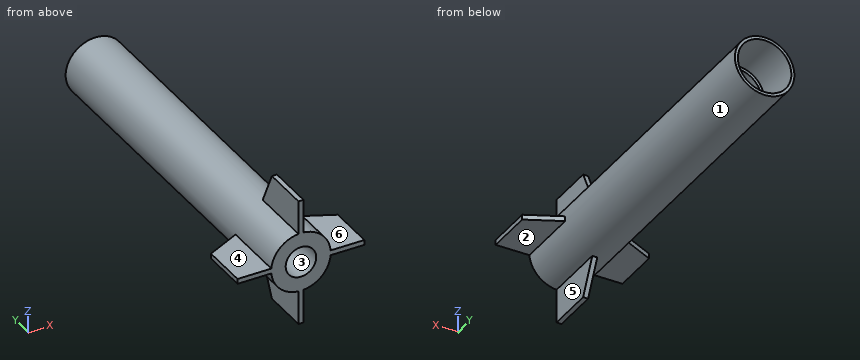
```python
from build123d import *

# Parameters (mm, degrees)
SKETCH1_R                = 11.925
SKETCH1_R_2              = 9.525
BOSS_EXTRUDE1_DEPTH      = 145
BOSS_EXTRUDE2_DEPTH      = 1
CIRPATTERN1_COUNT        = 4
SKETCH3_R                = 7.325
SKETCH3_R_2              = 6.125
BOSS_EXTRUDE3_DEPTH      = 87.75
CUT_EXTRUDE1_START       = -19
SKETCH4_R                = 10.725
SKETCH4_R_2              = 9.525
CUT_EXTRUDE1_DEPTH       = 19
BOSS_EXTRUDE4_START      = -1
SKETCH5_R                = 9.525
SKETCH5_R_2              = 6.125
BOSS_EXTRUDE4_DEPTH      = 1
BOSS_EXTRUDE5_DEPTH      = 0.5
BOSS_EXTRUDE5_DEPTH_BACK = 0.5
SKETCH6_R                = 9.525
SKETCH6_R_2              = 6.125
SKETCH7_R                = 9.525
SKETCH7_R_2              = 6.125
BOSS_EXTRUDE6_DEPTH      = 1


with BuildPart() as part:
    # Sketch1 → Boss-Extrude1 (new body)
    with BuildSketch(Plane(origin=(0, 0, 0), x_dir=(1, 0, 0), z_dir=(0, 1, 0))):
        with Locations(Location((0, 0, 0), (0, 0, 270))):
            Circle(SKETCH1_R)
        with Locations(Location((0, 0, 0), (0, 0, 270))):
            Circle(SKETCH1_R_2, mode=Mode.SUBTRACT)
    extrude(amount=BOSS_EXTRUDE1_DEPTH)

    # Sketch2 → Boss-Extrude2 (add, symmetric)
    with BuildSketch(Plane.XY):
        Polygon((-9.525, 0), (-9.525, 0.375), (-6.397493745, 0.375), (-6.397493745, 25.875), (-9.525, 25.875), (-9.525, 26.25), (-9.780127693, 26.25), (-25.405127693, 18.75), (-25.405127693, 0), align=None)
    boss_extrude2 = extrude(amount=BOSS_EXTRUDE2_DEPTH, both=True)

    # CirPattern1: Boss-Extrude2 ×4 about axis
    cirpattern1_axis = Axis((0, 0, 0), (0, 1, 0))
    for i in range(1, CIRPATTERN1_COUNT):
        add(boss_extrude2.rotate(cirpattern1_axis, i * 360 / CIRPATTERN1_COUNT))

    # Sketch4 → Cut-Extrude1 (cut)
    with BuildSketch(Plane(origin=(0, 145, 0), x_dir=(1, 0, 0), z_dir=(0, 1, 0)).offset(CUT_EXTRUDE1_START)):
        with Locations(Location((0, 0, 0), (0, 0, 270))):
            Circle(SKETCH4_R)
        with Locations(Location((0, 0, 0), (0, 0, 270))):
            Circle(SKETCH4_R_2, mode=Mode.SUBTRACT)
    extrude(amount=CUT_EXTRUDE1_DEPTH, mode=Mode.SUBTRACT)



with BuildPart() as body_2:
    # Sketch3 → Boss-Extrude3 (new body)
    with BuildSketch(Plane.XZ):
        with Locations(Location((0, 0, 0), (0, 0, 270))):
            Circle(SKETCH3_R)
        with Locations(Location((0, 0, 0), (0, 0, 270))):
            Circle(SKETCH3_R_2, mode=Mode.SUBTRACT)
    extrude(amount=-BOSS_EXTRUDE3_DEPTH)


with BuildPart() as part_1:
    add(part.part)

    add(body_2.part)  # Boss-Extrude4 merges body 2
    # Sketch5 → Boss-Extrude4 (add)
    with BuildSketch(Plane(origin=(0, 87.75, 0), x_dir=(1, 0, 0), z_dir=(0, 1, 0)).offset(BOSS_EXTRUDE4_START)):
        with Locations(Location((0, 0, 0), (0, 0, 90))):
            Circle(SKETCH5_R)
        with Locations(Location((0, 0, 0), (0, 0, 90))):
            Circle(SKETCH5_R_2, mode=Mode.SUBTRACT)
    extrude(amount=BOSS_EXTRUDE4_DEPTH)

    # Sketch6 → Boss-Extrude5 (add, two sides: drawn at the far end of the back side and taken through both)
    with BuildSketch(Plane(origin=(0, 43.875, 0), x_dir=(1, 0, 0), z_dir=(0, 1, 0)).offset(-BOSS_EXTRUDE5_DEPTH_BACK)):
        with Locations(Location((0, 0, 0), (0, 0, 270))):
            Circle(SKETCH6_R)
        with Locations(Location((0, 0, 0), (0, 0, 90))):
            Circle(SKETCH6_R_2, mode=Mode.SUBTRACT)
    extrude(amount=BOSS_EXTRUDE5_DEPTH + BOSS_EXTRUDE5_DEPTH_BACK)

    # Sketch7 → Boss-Extrude6 (add)
    with BuildSketch(Plane.XZ):
        with Locations(Location((0, 0, 0), (0, 0, 270))):
            Circle(SKETCH7_R)
        with Locations(Location((0, 0, 0), (0, 0, 270))):
            Circle(SKETCH7_R_2, mode=Mode.SUBTRACT)
    extrude(amount=-BOSS_EXTRUDE6_DEPTH)


solid = part_1.part
```
Geometry check sheet. Reference: the model listing, model coordinates, mm. Face numbers are marked on the shaded views. A direction names the side the tool comes from. Round coordinates to 2 decimals unless told otherwise and drop trailing zeros. Order: outer loops, then holes, each group sorted by start corner. A loop starts at its lowest first (then second) coordinate and runs counter-clockwise, first axis right, second up. Notation, with made-up numbers: M 81,-14.5 L 101,-14.5 A15 cw 101,5.5 Z; hole C -35.75,12.5 d11. An arc over 180 degrees is marked long. Write item = value, one per line.
Q1. Section check C-C (x = 21.5). Enter the section's corners in (y, z).
Answer block:
outline = M 0,-1 L 20.62,-1 L 20.62,1 L 0,1 Z
Q2. Section check B-B (y = 107.5). Enter the section's corners in (x, z) (3 decimals).
Answer block:
outline = C 0,0 d23.85; hole C 0,0 d19.05
Q3. Depth check by flat-ended pin: pin 1 Ø1.8 at (x, y) = (9, 10.5) entering from +Z; pin 2 Ø10 at (x, y) = (4.5, 74) entering from -Z (3 decimals); pin 3 Ø1.8 at (y, z) = (15.5, -9) entering from +X; pin 4 Ø10 at (y, z) = (123.5, -19) entering from -X. Enter the tip coordinate at first touch or a pass-through.
Answer block:
pin_1 = 8.75
pin_2 = -11.925
pin_3 = 8.75
pin_4 = through
Q4. Release check for a two-part mould opening along Z. For the marked faces 1, 2 and 3 record: released by +Z, released by -Z, zero draft, split by the parting line, or undercut.
Answer block:
face_1 = split by the parting line
face_2 = released by -Z
face_3 = undercut
Q5. Set-up check for the marked faces 4, 5 and 6: record each of +Z, -Z, +X, -X, +Y, -Y from which the full face is reachable in a straight line by a thin tool's end or side.
Answer block:
face_4 = +Z, -X, +Y, -Y
face_5 = -Z, +X, +Y, -Y
face_6 = +Z, +X, +Y, -Y
Q6. Section check A-A (y = 38.5). Enter the section's corners in (x, z) (3 decimals).
Answer block:
outline = C 0,0 d23.85; C 0,0 d14.65; hole C 0,0 d19.05; hole C 0,0 d12.25
Q7. Section check D-D (z = 17). Enter the section's corners in (x, y).
Answer block:
outline = M -1,0 L 1,0 L 1,22.78 L -1,22.78 Z
Q8. Scan lines: line 1 (X direction, y = 62, z = 0) (3 decimals); line 2 (Z direction, x = -0.5, y = 40); line 3 (Y direction, x = -3, z = 7) (3 decimals). Record each from-to range of solid material in increasing order.
Answer block:
line_1 = -11.925 to -9.525, -7.325 to -6.125, 6.125 to 7.325, 9.525 to 11.925
line_2 = -11.91 to -9.51, -7.31 to -6.1, 6.1 to 7.31, 9.51 to 11.91
line_3 = 0 to 1, 43.375 to 44.375, 86.75 to 87.75
